```python
from build123d import *

# Parameters (mm, degrees)
SKETCH1_R           = 47.25
SKETCH1_R_2         = 2.5
BOSS_EXTRUDE1_DEPTH = 15


with BuildPart() as part:
    # Sketch1 → Boss-Extrude1 (new body)
    with BuildSketch(Plane(origin=(0, 0, 0), x_dir=(1, 0, 0), z_dir=(0, 1, 0))):
        Circle(SKETCH1_R)
        with Locations((0, 41.25)):
            Circle(SKETCH1_R_2, mode=Mode.SUBTRACT)
        with Locations((41.25, 0)):
            Circle(SKETCH1_R_2, mode=Mode.SUBTRACT)
        with Locations((0, -41.25)):
            Circle(SKETCH1_R_2, mode=Mode.SUBTRACT)
        with Locations((-41.25, 0)):
            Circle(SKETCH1_R_2, mode=Mode.SUBTRACT)
        with BuildLine():
            Line((-5, 18.589311445), (-5, 29.25))
            Line((-5, 29.25), (5, 29.25))
            Line((5, 29.25), (5, 18.589311445))
            ThreePointArc((5, 18.589311445), (0, -19.25), (-5, 18.589311445))
        make_face(mode=Mode.SUBTRACT)
    extrude(amount=BOSS_EXTRUDE1_DEPTH)


solid = part.part
```
Model file for the job. Use its own axes, mm. A direction names the side the tool comes from. Coordinates: 2 decimals unless noted, no trailing zeros. Write each loop counter-clockwise with the first axis right and the second up, starting at its lowest first coordinate (ties: lowest second). Pieces come first, ordered by that corner, then holes. Notation, with made-up numbers: (60.5, 60) - (97.5, 60) arc R28 cw to (97.5, 88) - close; hole circle Ø2 at (30, -1). An arc over 180 degrees is marked (long way). Use a Markdown table: item, result. Add a question column.
Item 1: Band-saw the part on D-D, the plane z = -41.25. Write the cut outline in (x, y).
Item 2: Band-saw the part on A-A, the plane x = 0. Write the cut outline in (y, z).
Item 3: 3-axis set-ups, long thin cutter, end or side, ignore diameter. For faces 4 (the face through (-1, 15, 20)), 5 (the face through (0, 7, -29.25)): which of +Z, -Z, +X, -X, +Y, -Y reach the whole face in a straight line?
Item 4: Drill centre lines: line 1 along X through (y, z) = (6.5, 0); line 2 along X through (y, z) = (12, -41.25); line 3 along Z through (x, y) = (-14.5, 4.5). Where is each one in solid material? Low to high.
Item 5: Two-plate mould, pull along X, no slides. Class faces 1 (the face through (-37.496, 7.395, 28.751)), 2 (the face through (-0.5, 7.4, -38.8)), 3 (the face through (-1, 0, 20)): pulls with the +X half, pulls with the -X half, needs draft (parallel to the pull), parting line crosses it, or undercut.
Item 6: Band-saw the part on B-B, the plane z = 0. Write the cut outline in (x, y).
Item 7: Band-saw the part on C-C, the plane y = 12. Write the cut outline in (x, z).
Item 8: Drop flat-ended pins along their axis: pin 1 (5.5 mm diameter, centred on y = 5.5, z = -23.5, fed in from +X); pin 2 (4 mm diameter, centred on y = 1.5, z = 20, fed in from +X); pin 3 (3 mm diameter, centred on y = 7, z = -26.5, fed in from -X). Give the stop position or say it passes through.
A:
| question | item | result |
|---|---|---|
| 1 | outline | (-23.04, 0) - (-2.5, 0) - (-2.5, 15) - (-23.04, 15) - close; (2.5, 0) - (23.04, 0) - (23.04, 15) - (2.5, 15) - close |
| 2 | outline | (0, -47.25) - (15, -47.25) - (15, -43.75) - (0, -43.75) - close; (0, -38.75) - (15, -38.75) - (15, -29.25) - (0, -29.25) - close; (0, 19.25) - (15, 19.25) - (15, 38.75) - (0, 38.75) - close; (0, 43.75) - (15, 43.75) - (15, 47.25) - (0, 47.25) - close |
| 3 | face 4 | +Z, -Z, +X, -X, +Y |
| 3 | face 5 | +Y, -Y |
| 4 | line 1 | x = -47.25 to -43.75, -38.75 to -19.25, 19.25 to 38.75, 43.75 to 47.25 |
| 4 | line 2 | x = -23.04 to -2.5, 2.5 to 23.04 |
| 4 | line 3 | z = -44.97 to -12.66, 12.66 to 44.97 |
| 5 | face 1 | parting line crosses it |
| 5 | face 2 | undercut |
| 5 | face 3 | needs draft |
| 6 | outline | (-47.25, 0) - (-43.75, 0) - (-43.75, 15) - (-47.25, 15) - close; (-38.75, 0) - (-19.25, 0) - (-19.25, 15) - (-38.75, 15) - close; (19.25, 0) - (38.75, 0) - (38.75, 15) - (19.25, 15) - close; (43.75, 0) - (47.25, 0) - (47.25, 15) - (43.75, 15) - close |
| 7 | outline | circle Ø94.5 at (0, 0); hole circle Ø5 at (-41.25, 0); hole (-5, -29.25) - (5, -29.25) - (5, -18.59) arc R19.25 ccw (long way) to (-5, -18.59) - close; hole circle Ø5 at (0, -41.25); hole circle Ø5 at (0, 41.25); hole circle Ø5 at (41.25, 0) |
| 8 | pin 1 | stops at x = 42.45 |
| 8 | pin 2 | stops at x = 43.69 |
| 8 | pin 3 | stops at x = -40.09 |
